The listing builds one solid part. Answer for the finished solid, in the listing's coordinates (mm). Face numbers are marked on the shaded views. A direction names the side the tool comes from. Coordinates: 2 decimals unless noted, no trailing zeros. Order: outer loops, then holes, each group sorted by start corner. A loop starts at its lowest first (then second) coordinate and runs counter-clockwise, first axis right, second up. Notation, with made-up numbers: (-5.5, 61) -> (12.5, 61) arc R12 cw to (12.5, 81) -> close; hole circle Ø2 at (19, -16.5). An arc over 180 degrees is marked (long way). Write item = value, one per line. Start each with the question number.
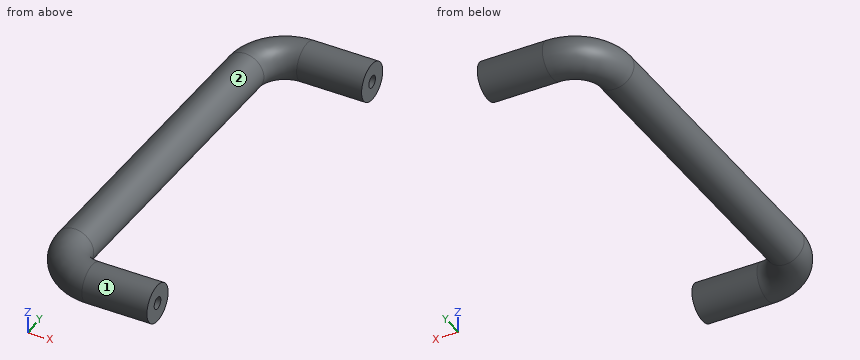
```python
from build123d import *

# Parameters (mm, degrees)
ESBO_O2_R             = 4.75
ESBO_O3_R             = 1.5
CORTE_EXTRUS_O1_DEPTH = 10


with BuildPart() as part:
    # Varredura1: sweep along a path in Esboço1
    with BuildLine(Plane.XY) as varredura1_path:
        Line((0, 0), (-16.25, 0))
        ThreePointArc((-16.25, 0), (-23.321067812, -2.928932188), (-26.25, -10))
        Line((-26.25, -10), (-26.25, -86.5))
        ThreePointArc((-26.25, -86.5), (-23.321067812, -93.571067812), (-16.25, -96.5))
        Line((-16.25, -96.5), (0, -96.5))
    # Esboço2 → Varredura1 (sweep)
    with BuildSketch(Plane(origin=(0, 0, 0), x_dir=(0, 0, -1), z_dir=(1, 0, 0))):
        Circle(ESBO_O2_R)
    sweep(path=varredura1_path.line)

    # Esboço3 → Corte-extrusão1 (cut)
    with BuildSketch(Plane(origin=(0, 0, 0), x_dir=(0, 0, -1), z_dir=(1, 0, 0))):
        Circle(ESBO_O3_R)
        with Locations((0, -96.5)):
            Circle(ESBO_O3_R)
    extrude(amount=-CORTE_EXTRUS_O1_DEPTH, mode=Mode.SUBTRACT)


solid = part.part
```
Item 1: Section A-A, the plane z = 0 is taken. Give the vertices of the cut face in (x, y), then the cut area to 3 significant figures.
Item 2: Consider probe 1 along Y at (x, z) = (-1.75, 0); probe 2 along Y at (x, z) = (-7, 1.25); probe 3 along Y at (x, z) = (-13.5, -2.75). Determine where each line is inside the solid, lowest interval first.
Item 3: Which of the six approach directions +Z, -Z, +X, -X, +Y, -Y give full straight-line access (tool end or side, diameter ignored) to the marked faces 1 and 2?
Item 4: Section B-B, the plane y = -77 is taken. Give the vertices of the cut face in (x, z).
Item 5: Each of these flat-tipped pins is pushed along its axis until it touches: pin 1 (2 mm diameter, centred on y = -11.5, z = 0.5, fed in from -X); pin 2 (4 mm diameter, centred on x = -10.5, z = -3.5, fed in from -Y); pin 3 (0.9 mm diameter, centred on y = -96, z = -0.5, fed in from +X); pin 4 (4 mm diameter, centred on x = -19.5, z = 1.5, fed in from -Y). Where does it stop, or does it pass through?
A:
q1.outline = (-31, -86.5) arc R14.75 ccw to (-16.25, -101.25) -> (0, -101.25) -> (0, -98) -> (-10, -98) -> (-10, -95) -> (0, -95) -> (0, -91.75) -> (-16.25, -91.75) arc R5.25 cw to (-21.5, -86.5) -> (-21.5, -10) arc R5.25 cw to (-16.25, -4.75) -> (0, -4.75) -> (0, -1.5) -> (-10, -1.5) -> (-10, 1.5) -> (0, 1.5) -> (0, 4.75) -> (-16.25, 4.75) arc R14.75 ccw to (-31, -10) -> close
q1.area = 1,270 mm^2
q2.probe_1 = -101.25 to -98, -95 to -91.75, -4.75 to -1.5, 1.5 to 4.75
q2.probe_2 = -101.08 to -97.33, -95.67 to -91.92, -4.58 to -0.83, 0.83 to 4.58
q2.probe_3 = -100.37 to -92.63, -3.87 to 3.87
q3.face_1 = +X
q3.face_2 = none
q4.outline = circle Ø9.5 at (-26.25, 0)
q5.pin_1 = -31
q5.pin_2 = -101.01
q5.pin_3 = -10
q5.pin_4 = -101.15
